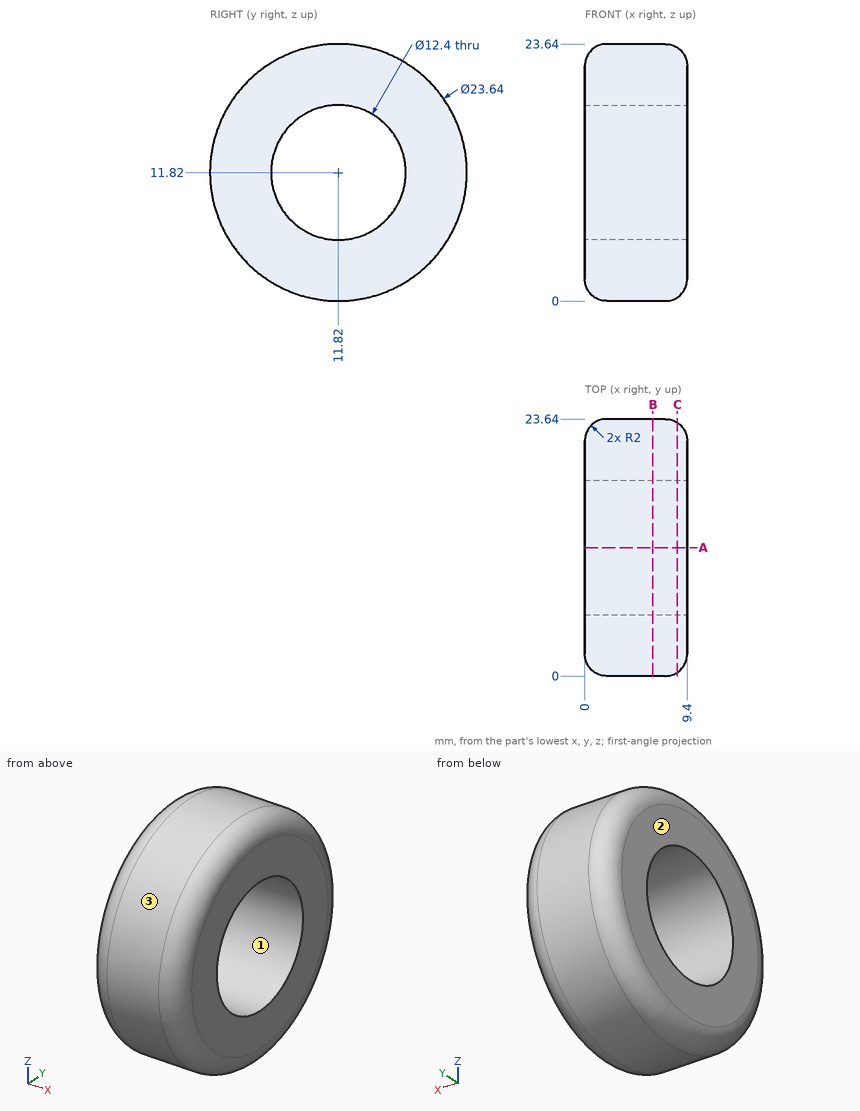
Drawing for the job (mm, zero at the part's lowest x, y, z). Round coordinates to 2 decimals unless told otherwise and drop trailing zeros. Loops run counter-clockwise (first coordinate to the right, second up) from the corner with the lowest first, then second, coordinate; pieces in that order, holes last. Notation, with made-up numbers: (70.5, -23.5) -> (122.5, -23.5) arc R24 ccw to (122.5, -5.5) -> close; hole circle Ø5 at (36.25, 79.5). An arc over 180 degrees is marked (long way). Use one line per item in the form item = value. Start each with the question number.
Item 1: Drop flat-ended pins along their axis: pin 1 Ø1.5 at (x, z) = (3, 19) entering from +Y; pin 2 Ø11 at (y, z) = (11.82, 11.82) entering from +X; pin 3 Ø1.5 at (x, y) = (6.5, 21) entering from -Z; pin 4 Ø1 at (x, y) = (7, 9.5) entering from -Z. Give the stop position or say it passes through.
Item 2: Band-saw the part on C-C (x = 8.5). List the corners of the cut face in (y, z).
Item 3: Drill centre lines: line 1 along Y through (x, z) = (5, 11.82); line 2 along Y through (x, z) = (7.5, 6.25); line 3 along Z through (x, y) = (1.25, 14.25). Where is each one in solid material? Low to high.
Item 4: Band-saw the part on B-B (x = 6.25). List the corners of the cut face in (y, z), plus the area to 3 significant figures.
Item 5: Two-plate mould, pull along Y, no slides. Class the marked faces 1, 2 and 3: released by +Y, released by -Y, zero draft, split by the parting line, or undercut.
Item 6: Band-saw the part on A-A (y = 11.82). List the corners of the cut face in (x, z), plus the area to 3 significant figures.
Data:
q1.pin_1 = 21.74
q1.pin_2 = through
q1.pin_3 = 3.53
q1.pin_4 = 0.14
q2.outline = circle Ø22.98 at (11.82, 11.82); hole circle Ø12.4 at (11.82, 11.82)
q3.line_1 = 0 to 5.62, 18.02 to 23.64
q3.line_2 = 1.4 to 9.1, 14.54 to 22.24
q3.line_3 = 0.4 to 6.12, 17.52 to 23.24
q4.outline = circle Ø23.64 at (11.82, 11.82); hole circle Ø12.4 at (11.82, 11.82)
q4.area = 318 mm^2
q5.face_1 = undercut
q5.face_2 = zero draft
q5.face_3 = split by the parting line
q6.outline = (0, 2) arc R2 ccw to (2, 0) -> (7.4, 0) arc R2 ccw to (9.4, 2) -> (9.4, 5.62) -> (0, 5.62) -> close; (0, 18.02) -> (9.4, 18.02) -> (9.4, 21.64) arc R2 ccw to (7.4, 23.64) -> (2, 23.64) arc R2 ccw to (0, 21.64) -> close
q6.area = 102 mm^2
